CAD build for the part. Positions are in the model's coordinates, mm. Coordinates: 2 decimals unless noted, no trailing zeros. Loops run counter-clockwise (first coordinate to the right, second up) from the corner with the lowest first, then second, coordinate; pieces in that order, holes last. Notation, with made-up numbers: (56.25, 23) -> (97.25, 23) arc R23 cw to (97.25, 34) -> close; hole circle Ø11 at (87.5, -21). An arc over 180 degrees is marked (long way). Return JSON: item names as keys, results as strings. Group by question number.
(1) Probe L1, parallel to Y at x = 11, z = 1.35; L2, parallel to Y at x = 12, z = 0.35; L3, parallel to Y at x = -42, z = 0.85. List the from-to ranges inside material, lowest first.
(2) Saw through at D-D on x = 5.5. Write the cut outline in (y, z), then the cut area to 3 significant figures.
(3) Saw through at B-B on x = -50. Write the cut outline in (y, z).
(4) Saw through at A-A on y = 0. Write the cut outline in (x, z).
(5) Saw through at C-C on z = 0.95. Write the cut outline in (x, y).
(6) Flat gauge pins, fed straight in: pin 1 Ø1 at (x, z) = (-41, 1) entering from -Y; pin 2 Ø8.5 at (x, y) = (11, 20) entering from +Z. Where does each tip first touch, or does it go through?
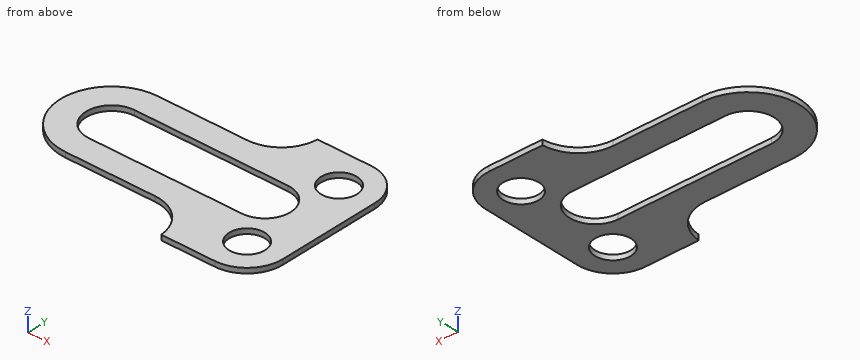
```python
from build123d import *

# Parameters (mm, degrees)
SKETCH_R  = 7
PAD_DEPTH = 2


with BuildPart() as part:
    # Sketch → Pad (new body)
    with BuildSketch(Plane.XY):
        with BuildLine():
            Line((-10, 34), (11, 34))
            ThreePointArc((25, 20), (20.899495, 29.899495), (11, 34))
            Line((25, 20), (25, -20))
            ThreePointArc((11, -34), (20.899495, -29.899495), (25, -20))
            Line((11, -34), (-10, -34))
            ThreePointArc((-10, -34), (-14.719679, -24.045549), (-24.96663, -20))
            Line((-24.96663, -20), (-60.000002, -20))
            ThreePointArc((-60.000002, 20), (-80, 0), (-60.000002, -20))
            Line((-60.000002, 20), (-24.96663, 20))
            ThreePointArc((-24.96663, 20), (-14.719679, 24.045549), (-10, 34))
        make_face()
        with Locations((11, 20)):
            Circle(SKETCH_R, mode=Mode.SUBTRACT)
        with Locations((11, -20)):
            Circle(SKETCH_R, mode=Mode.SUBTRACT)
        with BuildLine():
            ThreePointArc((-60.000002, 10), (-70, 0), (-60.000002, -10))
            Line((-60.000002, -10), (0, -10))
            ThreePointArc((0, -10), (10, 0), (0, 10))
            Line((-60.000002, 10), (0, 10))
        make_face(mode=Mode.SUBTRACT)
    extrude(amount=PAD_DEPTH)


solid = part.part
```
Geometry results:
{
 "1": {"L1": "-34 to -27, -13 to 13, 27 to 34", "L2": "-33.96 to -26.93, -13.07 to 13.07, 26.93 to 33.96", "L3": "-20 to -10, 10 to 20"},
 "2": {"outline": "(-34, 0) -> (-24.33, 0) -> (-24.33, 2) -> (-34, 2) -> close; (-15.67, 0) -> (-8.35, 0) -> (-8.35, 2) -> (-15.67, 2) -> close; (8.35, 0) -> (15.67, 0) -> (15.67, 2) -> (8.35, 2) -> close; (24.33, 0) -> (34, 0) -> (34, 2) -> (24.33, 2) -> close", "area": "68.0 mm²"},
 "3": {"outline": "(-20, 0) -> (-10, 0) -> (-10, 2) -> (-20, 2) -> close; (10, 0) -> (20, 0) -> (20, 2) -> (10, 2) -> close"},
 "4": {"outline": "(-80, 0) -> (-70, 0) -> (-70, 2) -> (-80, 2) -> close; (10, 0) -> (25, 0) -> (25, 2) -> (10, 2) -> close"},
 "5": {"outline": "(-60, -20) -> (-24.97, -20) arc R15 cw to (-10, -34) -> (11, -34) arc R14 ccw to (25, -20) -> (25, 20) arc R14 ccw to (11, 34) -> (-10, 34) arc R15 cw to (-24.97, 20) -> (-60, 20) arc R20 ccw to start; hole (-60, -10) -> (0, -10) arc R10 ccw to (0, 10) -> (-60, 10) arc R10 ccw to start; hole circle Ø14 at (11, -20); hole circle Ø14 at (11, 20)"},
 "6": {"pin 1": "y = -20", "pin 2": "through"}
}
